Source: CAD feature listing. Evaluate the final solid. Frame: model axes, mm. A direction names the side the tool comes from. Give positions to 0.01 mm unless a question says otherwise; leave off trailing zeros. Loops run counter-clockwise (first coordinate to the right, second up) from the corner with the lowest first, then second, coordinate; pieces in that order, holes last. Notation, with made-up numbers: M 6,-2 L 44,-2 A16 cw 44,13 Z; hole C 43,-7 d1. An arc over 180 degrees is marked long. Write item = value, one per line.
from build123d import *

# Parameters (mm, degrees)
SKETCH_1_W          = 33
SKETCH_1_H          = 10
SKETCH_1_R          = 2.025
EXTRUDE_1_DEPTH     = 10
CUT_EXTRUDE_1_DEPTH = 25
FILLET_1_R          = 1.5
FILLET_2_R          = 3


with BuildPart() as part:
    # 草图1 → 凸台-拉伸1 (new, symmetric)
    with BuildSketch(Plane.XY):
        Rectangle(SKETCH_1_W, SKETCH_1_H)
        with Locations((12.5, 0)):
            Circle(SKETCH_1_R, mode=Mode.SUBTRACT)
        with Locations(Location((-12.5, 0, 0), (0, 0, 180))):
            Circle(SKETCH_1_R, mode=Mode.SUBTRACT)
    extrude(amount=EXTRUDE_1_DEPTH, both=True)

    # 草图2 → 切除-拉伸1 (cut, symmetric)
    with BuildSketch(Plane.XY.offset(10)):
        with BuildLine():
            Line((-7.018154964, 2.5), (7.018154964, 2.5))
            ThreePointArc((7.018154964, 2.5), (6.475, 0), (7.018154964, -2.5))
            Line((7.018154964, -2.5), (-7.018154964, -2.5))
            ThreePointArc((-7.018154964, -2.5), (-6.475, 0), (-7.018154964, 2.5))
        make_face()
    extrude(amount=CUT_EXTRUDE_1_DEPTH, both=True, mode=Mode.SUBTRACT)

    # 圆角1
    fillet_1_edges = [part.edges().sort_by_distance(p)[0] for p in [
        (-7.018154964, -2.5, 0),
        (-7.018154964, 2.5, 0),
        (7.018154964, 2.5, 0),
        (7.018154964, -2.5, 0),
    ]]
    fillet(fillet_1_edges, radius=FILLET_1_R)

    # 圆角2
    fillet_2_edges = [part.edges().sort_by_distance(p)[0] for p in [
        (16.5, -5, 0),
        (-16.5, -5, 0),
        (-16.5, 5, 0),
        (16.5, 5, 0),
    ]]
    fillet(fillet_2_edges, radius=FILLET_2_R)


solid = part.part
1. Reachability of faces 4 (the cylindrical face through (-15.64, 4.1, -0.14)), 5 (the cylindrical face through (-6.182, 1.974, 0.14)) from +Z, -Z, +X, -X, +Y, -Y: full face, straight path, thin tool, end or side. Return the list, or none.
Derived:
face_4 = +Z, -Z, -X, +Y
face_5 = +Z, -Z
2. Cut plane C-C, the plane y = 0. Return the cut outline in (x, z) (3 decimals).
Derived:
outline = M -16.5,-10 L -14.525,-10 L -14.525,10 L -16.5,10 Z; M -10.475,-10 L -6.475,-10 L -6.475,10 L -10.475,10 Z; M 6.475,-10 L 10.475,-10 L 10.475,10 L 6.475,10 Z; M 14.525,-10 L 16.5,-10 L 16.5,10 L 14.525,10 Z
3. Material intervals for probe 1 along Y at (x, z) = (-12.5, -2) (3 decimals); probe 2 along X at (y, z) = (1, -8.5); probe 3 along Y at (x, z) = (-1.5, 1.25), sorted ascending. Write a range as from..to.
Derived:
probe_1 = -5..-2.025, 2.025..5
probe_2 = -16.5..-14.26, -10.74..-6.54, 6.54..10.74, 14.26..16.5
probe_3 = -5..-2.5, 2.5..5
4. Cut plane B-B, the plane x = -1. Return the cut outline in (y, z).
Derived:
outline = M -5,-10 L -2.5,-10 L -2.5,10 L -5,10 Z; M 2.5,-10 L 5,-10 L 5,10 L 2.5,10 Z
5. Cut plane D-D, the plane x = 12.5. Return the cut outline in (y, z) (3 decimals).
Derived:
outline = M -5,-10 L -2.025,-10 L -2.025,10 L -5,10 Z; M 2.025,-10 L 5,-10 L 5,10 L 2.025,10 Z
6. Pull-direction query (Y, two-part tool) for faces 1 (the cylindrical face through (6.182, 1.974, -0.14)), 2 (the flat face through (0, 3, -10)), 3 (the flat face through (0, -5, 0)); classes: +Y half, -Y half, draft (parallel to the pull), parting line (faces both ways), or undercut.
Derived:
face_1 = undercut
face_2 = draft
face_3 = -Y half
7. Cut plane A-A, the plane z = -1.5. Return the cut outline in (x, y) (3 decimals).
Derived:
outline = M -16.5,-2 A3 ccw -13.5,-5 L 13.5,-5 A3 ccw 16.5,-2 L 16.5,2 A3 ccw 13.5,5 L -13.5,5 A3 ccw -16.5,2 Z; hole C -12.5,0 d4.05; hole M -6.528,-0.801 A1.5 ccw -5.042,-2.5 L 5.042,-2.5 A1.5 ccw 6.528,-0.801 A6.025 cw 6.528,0.801 A1.5 ccw 5.042,2.5 L -5.042,2.5 A1.5 ccw -6.528,0.801 A6.025 cw Z; hole C 12.5,0 d4.05
